For this review, take the finished solid that the model builds, in its own axes (mm). A direction names the side the tool comes from. Round coordinates to 2 decimals unless told otherwise and drop trailing zeros. Loops run counter-clockwise (first coordinate to the right, second up) from the corner with the lowest first, then second, coordinate; pieces in that order, holes last.
```python
from build123d import *

# Parameters (mm, degrees)
SKETCH1_W           = 79.809734904
SKETCH1_H           = 42.557787138
BOSS_EXTRUDE1_DEPTH = 2.7


with BuildPart() as part:
    # Sketch1 → Boss-Extrude1 (new body)
    with BuildSketch(Plane.XY):
        Rectangle(SKETCH1_W, SKETCH1_H)
        Polygon((-24.904867452, -0.928893569), (-0.190628486, 3.428893569), (24.904867452, 3.428893569), (24.904867452, 6.278893569), (-0.190628486, 6.278893569), (-0.685525793, 6.235595665), (-25.399764759, 1.877808527), align=None, mode=Mode.SUBTRACT)
        Polygon((-24.904867452, -3.428893569), (0.190628486, -3.428893569), (24.904867452, 0.928893569), (25.399764759, -1.877808527), (0.685525793, -6.235595665), (0.190628486, -6.278893569), (-24.904867452, -6.278893569), align=None, mode=Mode.SUBTRACT)
    extrude(amount=BOSS_EXTRUDE1_DEPTH)


solid = part.part
```
(1) Add section A-A (x = -12). Give the boundary of the cut face in (y, z).
(2) Insertion check: pin 1 Ø4 at (x, y) = (19, 8.5) entering from -Z. The pin has a flat end and moves straight along its axis. Give the tip position at first contact, or say it passes through.
(3) Add section B-B (z = 1). Give the boundary of the cut face in (x, y), plus the area to 3 significant figures.
(4) For faces 1 (the flat face through (-24.905, -5, 1)), 2 (the flat face through (-1, 21.279, 1)), list the 3-axis set-ups (+Z, -Z, +X, -X, +Y, -Y) from which the entire face can be reached by the end or side of a thin tool; tool diameter is ignored.
(5) The part is to be moulded in two halves that separate along X. For faces 3 (the flat face through (-12.72, 1.22, 1.33)), 4 (the flat face through (-39.905, 0, 1)), 5 (the flat face through (39.905, 0, 1)), 6 (the flat face through (13, 6.279, 1)), say which applies: pulls with the +X half, pulls with the -X half, needs draft (parallel to the pull), parting line crosses it, or undercut.
(6) Add section C-C (y = -4.5). Give the boundary of the cut face in (x, z), plus the area to 3 significant figures.
(7) For L1, parallel to Y at x = 4, z = 0.45; L2, parallel to Y at x = 18.5, z = 2, list the stretches that pass through material, from the lowest coordinate up.
Outcome:
1. outline: (-21.28, 0) - (-6.28, 0) - (-6.28, 2.7) - (-21.28, 2.7) - close; (-3.43, 0) - (1.35, 0) - (1.35, 2.7) - (-3.43, 2.7) - close; (4.24, 0) - (21.28, 0) - (21.28, 2.7) - (4.24, 2.7) - close
2. pin 1: stops at z = 0
3. outline: (-39.9, -21.28) - (39.9, -21.28) - (39.9, 21.28) - (-39.9, 21.28) - close; hole (-25.4, 1.88) - (-24.9, -0.93) - (-0.19, 3.43) - (24.9, 3.43) - (24.9, 6.28) - (-0.19, 6.28) - (-0.69, 6.24) - close; hole (-24.9, -6.28) - (0.19, -6.28) - (0.69, -6.24) - (25.4, -1.88) - (24.9, 0.93) - (0.19, -3.43) - (-24.9, -3.43) - close
3. area: 3,110 mm2
4. face 1: +Z, -Z
4. face 2: +Z, -Z, +X, -X, +Y
5. face 3: undercut
5. face 4: pulls with the -X half
5. face 5: pulls with the +X half
5. face 6: undercut
6. outline: (-39.9, 0) - (-24.9, 0) - (-24.9, 2.7) - (-39.9, 2.7) - close; (10.53, 0) - (39.9, 0) - (39.9, 2.7) - (10.53, 2.7) - close
6. area: 120 mm2
7. L1: y = -21.28 to -5.65, -2.76 to 3.43, 6.28 to 21.28
7. L2: y = -21.28 to -3.09, -0.2 to 3.43, 6.28 to 21.28
